Geometry check sheet. Reference: drawing and pictorial views, mm from the part's lowest x, y, z. Round coordinates to 2 decimals unless told otherwise and drop trailing zeros. Write each loop counter-clockwise with the first axis right and the second up, starting at its lowest first coordinate (ties: lowest second). Pieces come first, ordered by that corner, then holes. Notation, with made-up numbers: M -29,26.5 L 8,26.5 A24 cw 8,50.5 Z; hole C -36.5,-36 d10. An arc over 180 degrees is marked long. Use a Markdown table: item, result. Add a question column.
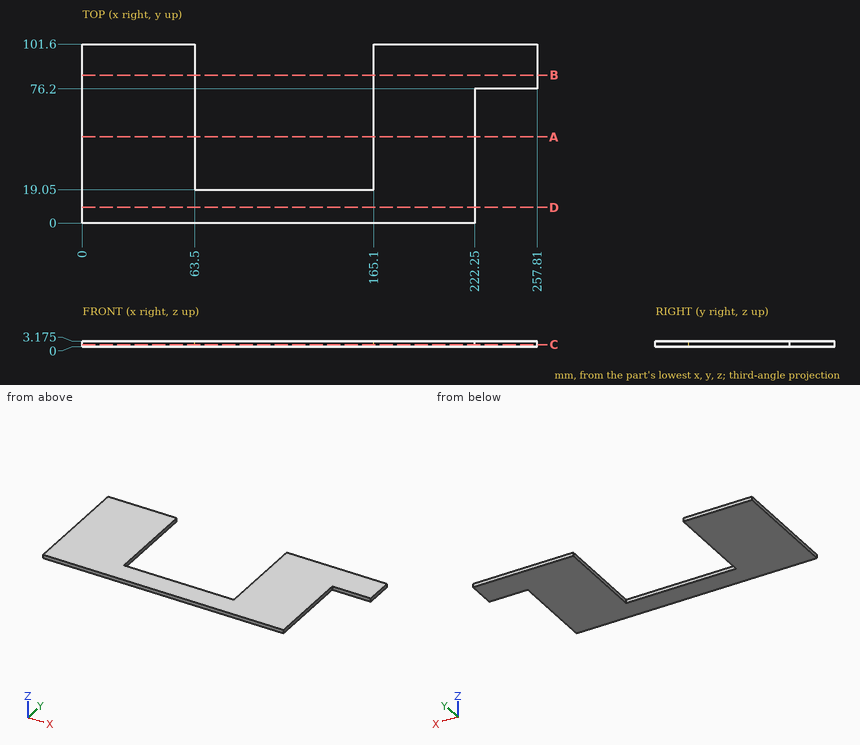
1. Cross-section at A-A on y = 49. Enter the section's corners in (x, z) (3 decimals).
2. Cross-section at B-B on y = 84. Enter the section's corners in (x, z) (3 decimals).
3. Scan lines: line 1 along X through (y, z) = (39, 1.8); line 2 along X through (y, z) = (87.5, 0.6); line 3 along Y through (x, z) = (101.5, 0.7). Record each from-to range of solid material in increasing order. Write a range as from..to.
4. Cross-section at D-D on y = 9. Enter the section's corners in (x, z) (3 decimals), plus the area to 3 significant figures.
5. Depth check by flat-ended pin: pin 1 Ø1.5 at (y, z) = (51.5, 2) entering from +X; pin 2 Ø1.6 at (x, z) = (128, 1) entering from +Y. Enter the tip coordinate at first touch or a pass-through.
6. Cross-section at C-C on z = 1.25. Enter the section's corners in (x, y), plus the area to 3 significant figures.
Answer:
| question | item | result |
|---|---|---|
| 1 | outline | M 0,0 L 63.5,0 L 63.5,3.175 L 0,3.175 Z; M 165.1,0 L 222.25,0 L 222.25,3.175 L 165.1,3.175 Z |
| 2 | outline | M 0,0 L 63.5,0 L 63.5,3.175 L 0,3.175 Z; M 165.1,0 L 257.81,0 L 257.81,3.175 L 165.1,3.175 Z |
| 3 | line 1 | x = 0..63.5, 165.1..222.25 |
| 3 | line 2 | x = 0..63.5, 165.1..257.81 |
| 3 | line 3 | y = 0..19.05 |
| 4 | outline | M 0,0 L 222.25,0 L 222.25,3.175 L 0,3.175 Z |
| 4 | area | 706 mm^2 |
| 5 | pin 1 | stops at x = 222.25 |
| 5 | pin 2 | stops at y = 19.05 |
| 6 | outline | M 0,0 L 222.25,0 L 222.25,76.2 L 257.81,76.2 L 257.81,101.6 L 165.1,101.6 L 165.1,19.05 L 63.5,19.05 L 63.5,101.6 L 0,101.6 Z |
| 6 | area | 15,100 mm^2 |
